Could you check a few things on this drawing? It's one solid part, dimensions in mm from its lowest x, y, z. A direction names the side the tool comes from. Give positions to 0.01 mm unless a question says otherwise; leave off trailing zeros. Loops run counter-clockwise (first coordinate to the right, second up) from the corner with the lowest first, then second, coordinate; pieces in that order, holes last. Notation, with made-up numbers: M 86,68.25 L 129,68.25 A18 ccw 129,83.25 Z; hole C 8.25,65.25 d10. An arc over 180 degrees is marked long. One line per item, written item: value. Start each with the question number.
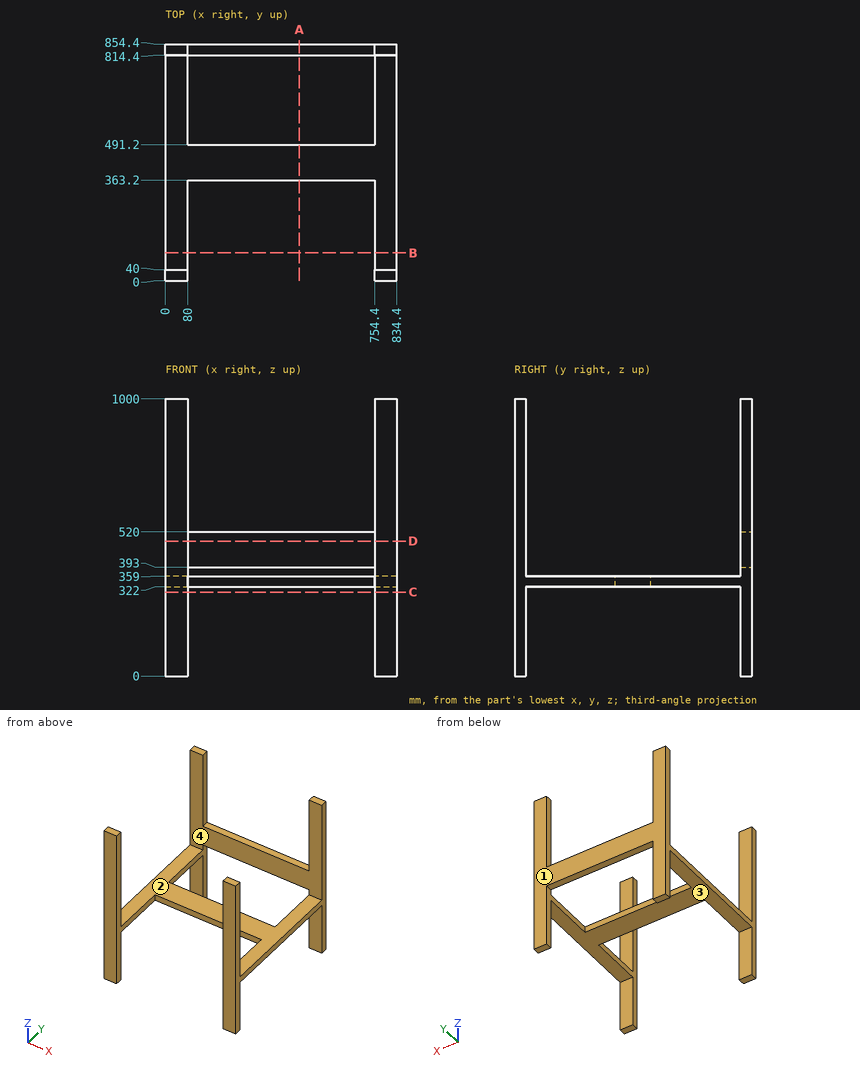
Q1. For P1, Ø2, axis at x = 112.5, y = 455, coming from the -Z side; P2, Ø20, axis at x = 431.5, y = 842, coming from the +Z side; P3, Ø12, axis at x = 277, y = 830, coming from the -Z side, each with a flat end and sliding along its axis, tell me the tip position at first contact or that it passes through.
Q2. I need wall thicknesses on line 1 along Z through (x, y) = (771, 261); line 2 along Y through (x, z) = (628.5, 443). Which ranges of each line are inside material? Lowest first, please.
Q3. Which directions (+Z, -Z, +X, -X, +Y, -Y) give clear straight access to the entire face, cutting with the end or side of a thin tool? Please do the marked faces 3 and 4.
Q4. If we section it at D-D, the plane z = 487: Write out the boundary of the cut face in (x, y), plus the area to 3 significant figures.
Q5. If we section it at B-B, the plane y = 100.5: Write out the boundary of the cut face in (x, z), plus the area to 3 significant figures.
Q6. If we section it at C-C, the plane z = 303: Write out the boundary of the cut face in (x, y).
Q7. If we mould it in two halves opening along Y, with no side actions, what happens to the marked faces 1 and 2? For each: released by +Y, released by -Y, zero draft, split by the parting line, or undercut.
Q8. If we section it at A-A, the plane x = 483.5: Write out the boundary of the cut face in (y, z), plus the area to 3 significant figures.
Response:
1. P1: z = 322
1. P2: z = 520
1. P3: z = 393
2. line 1: 322 to 359
2. line 2: 814.4 to 854.4
3. face 3: -Z, +X, -X
3. face 4: +Z, +X, -X
4. outline: M 0,0 L 80,0 L 80,40 L 0,40 Z; M 0,814.4 L 834.4,814.4 L 834.4,854.4 L 0,854.4 Z; M 754.4,0 L 834.4,0 L 834.4,40 L 754.4,40 Z
4. area: 39,800 mm^2
5. outline: M 0,322 L 80,322 L 80,359 L 0,359 Z; M 754.4,322 L 834.4,322 L 834.4,359 L 754.4,359 Z
5. area: 5,920 mm^2
6. outline: M 0,0 L 80,0 L 80,40 L 0,40 Z; M 0,814.4 L 80,814.4 L 80,854.4 L 0,854.4 Z; M 754.4,0 L 834.4,0 L 834.4,40 L 754.4,40 Z; M 754.4,814.4 L 834.4,814.4 L 834.4,854.4 L 754.4,854.4 Z
7. face 1: released by +Y
7. face 2: undercut
8. outline: M 363.2,322 L 491.2,322 L 491.2,359 L 363.2,359 Z; M 814.4,393 L 854.4,393 L 854.4,520 L 814.4,520 Z
8. area: 9,820 mm^2
